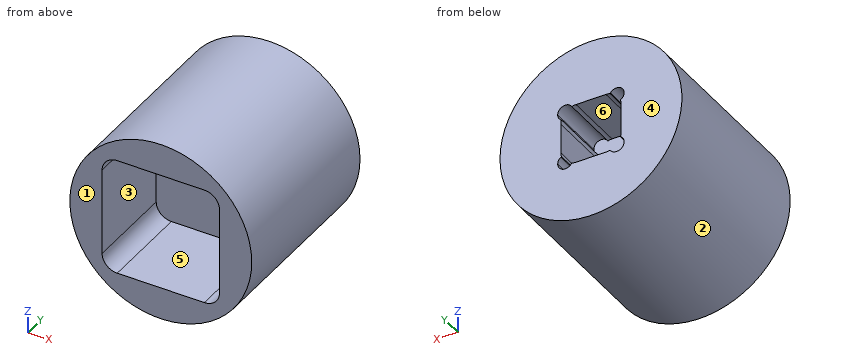
```python
from build123d import *

# Parameters (mm, degrees)
SKETCH1_R           = 19.05
BOSS_EXTRUDE1_DEPTH = 19.05
SKETCH2_W           = 12.6111
SKETCH2_H           = 12.6111
CUT_EXTRUDE1_DEPTH  = 12.7
CUT_EXTRUDE2_DEPTH  = 19.05
FILLET1_R           = 3.175
CUT_EXTRUDE3_DEPTH  = 12.7


with BuildPart() as part:
    # Sketch1 → Boss-Extrude1 (new body, symmetric)
    with BuildSketch(Plane(origin=(0, 0, 0), x_dir=(1, 0, 0), z_dir=(0, 1, 0))):
        Circle(SKETCH1_R)
    extrude(amount=BOSS_EXTRUDE1_DEPTH, both=True)

    # Sketch2 → Cut-Extrude1 (cut)
    with BuildSketch(Plane(origin=(0, 19.05, 0), x_dir=(1, 0, 0), z_dir=(0, 1, 0))):
        Rectangle(SKETCH2_W, SKETCH2_H)
    extrude(amount=-CUT_EXTRUDE1_DEPTH, mode=Mode.SUBTRACT)

    # Sketch3 → Cut-Extrude2 (cut)
    with BuildSketch(Plane.XZ.offset(19.05)):
        with BuildLine():
            Line((9.12495, 12.29995), (-9.12495, 12.29995))
            ThreePointArc((-9.12495, 12.29995), (-11.37001403, 11.37001403), (-12.29995, 9.12495))
            Line((-12.29995, 9.12495), (-12.29995, -9.12495))
            ThreePointArc((-12.29995, -9.12495), (-11.37001403, -11.37001403), (-9.12495, -12.29995))
            Line((-9.12495, -12.29995), (9.12495, -12.29995))
            ThreePointArc((9.12495, -12.29995), (11.37001403, -11.37001403), (12.29995, -9.12495))
            Line((12.29995, -9.12495), (12.29995, 9.12495))
            ThreePointArc((12.29995, 9.12495), (11.37001403, 11.37001403), (9.12495, 12.29995))
        make_face()
    extrude(amount=-CUT_EXTRUDE2_DEPTH, mode=Mode.SUBTRACT)

    # Fillet1
    fillet1_edges = [part.edges().sort_by_distance(p)[0] for p in [
        (-6.30555, 12.7, 6.30555),
        (-6.30555, 12.7, -6.30555),
        (6.30555, 12.7, -6.30555),
        (6.30555, 12.7, 6.30555),
    ]]
    fillet(fillet1_edges, radius=FILLET1_R)

    # Sketch4 → Cut-Extrude3 (cut)
    with BuildSketch(Plane(origin=(0, 19.05, 0), x_dir=(1, 0, 0), z_dir=(0, 1, 0))):
        with BuildLine():
            ThreePointArc((4.008094076, 6.181867977), (4.253082015, 4.253082015), (6.181867977, 4.008094076))
            ThreePointArc((6.181867977, 4.008094076), (5.37561403, 5.37561403), (4.008094076, 6.181867977))
        make_face()
        with BuildLine():
            ThreePointArc((6.181867977, 4.008094076), (6.244651028, 4.047106994), (6.30555, 4.089000125))
            Line((6.30555, 4.089000125), (6.30555, 6.30555))
            Line((6.30555, 6.30555), (4.089000125, 6.30555))
            ThreePointArc((4.089000125, 6.30555), (4.047106994, 6.244651028), (4.008094076, 6.181867977))
            ThreePointArc((4.008094076, 6.181867977), (5.37561403, 5.37561403), (6.181867977, 4.008094076))
        make_face()
        with BuildLine():
            Line((6.30555, 6.30555), (6.30555, 4.089000125))
            ThreePointArc((6.30555, 4.089000125), (6.789196289, 4.653158877), (6.96311403, 5.37561403))
            ThreePointArc((6.96311403, 5.37561403), (5.864314693, 6.886020569), (4.089000125, 6.30555))
            Line((4.089000125, 6.30555), (6.30555, 6.30555))
        make_face()
        with BuildLine():
            ThreePointArc((-4.008094076, 6.181867977), (-5.37561403, 5.37561403), (-6.181867977, 4.008094076))
            ThreePointArc((-6.181867977, 4.008094076), (-4.588140821, 3.997193849), (-3.78811403, 5.37561403))
            ThreePointArc((-3.78811403, 5.37561403), (-3.844096127, 5.793476641), (-4.008094076, 6.181867977))
        make_face()
        with BuildLine():
            Line((-6.30555, 6.30555), (-6.30555, 4.089000125))
            ThreePointArc((-6.30555, 4.089000125), (-6.244651028, 4.047106994), (-6.181867977, 4.008094076))
            ThreePointArc((-6.181867977, 4.008094076), (-5.37561403, 5.37561403), (-4.008094076, 6.181867977))
            ThreePointArc((-4.008094076, 6.181867977), (-4.047106994, 6.244651028), (-4.089000125, 6.30555))
            Line((-4.089000125, 6.30555), (-6.30555, 6.30555))
        make_face()
        with BuildLine():
            ThreePointArc((-4.089000125, 6.30555), (-6.498146045, 6.498146045), (-6.30555, 4.089000125))
            Line((-6.30555, 4.089000125), (-6.30555, 6.30555))
            Line((-6.30555, 6.30555), (-4.089000125, 6.30555))
        make_face()
        with BuildLine():
            ThreePointArc((-6.30555, -4.089000125), (-6.498146045, -6.498146045), (-4.089000125, -6.30555))
            Line((-4.089000125, -6.30555), (-6.30555, -6.30555))
            Line((-6.30555, -6.30555), (-6.30555, -4.089000125))
        make_face()
        with BuildLine():
            Line((-6.30555, -6.30555), (-4.089000125, -6.30555))
            ThreePointArc((-4.089000125, -6.30555), (-4.047106994, -6.244651028), (-4.008094076, -6.181867977))
            ThreePointArc((-4.008094076, -6.181867977), (-5.37561403, -5.37561403), (-6.181867977, -4.008094076))
            ThreePointArc((-6.181867977, -4.008094076), (-6.244651028, -4.047106994), (-6.30555, -4.089000125))
            Line((-6.30555, -4.089000125), (-6.30555, -6.30555))
        make_face()
        with BuildLine():
            ThreePointArc((-6.181867977, -4.008094076), (-5.37561403, -5.37561403), (-4.008094076, -6.181867977))
            ThreePointArc((-4.008094076, -6.181867977), (-3.844096127, -5.793476641), (-3.78811403, -5.37561403))
            ThreePointArc((-3.78811403, -5.37561403), (-4.588140821, -3.997193849), (-6.181867977, -4.008094076))
        make_face()
        with BuildLine():
            ThreePointArc((6.181867977, -4.008094076), (4.253082015, -4.253082015), (4.008094076, -6.181867977))
            ThreePointArc((4.008094076, -6.181867977), (5.37561403, -5.37561403), (6.181867977, -4.008094076))
        make_face()
        with BuildLine():
            ThreePointArc((4.008094076, -6.181867977), (4.047106994, -6.244651028), (4.089000125, -6.30555))
            Line((4.089000125, -6.30555), (6.30555, -6.30555))
            Line((6.30555, -6.30555), (6.30555, -4.089000125))
            ThreePointArc((6.30555, -4.089000125), (6.244651028, -4.047106994), (6.181867977, -4.008094076))
            ThreePointArc((6.181867977, -4.008094076), (5.37561403, -5.37561403), (4.008094076, -6.181867977))
        make_face()
        with BuildLine():
            Line((6.30555, -6.30555), (4.089000125, -6.30555))
            ThreePointArc((4.089000125, -6.30555), (5.864314693, -6.886020569), (6.96311403, -5.37561403))
            ThreePointArc((6.96311403, -5.37561403), (6.789196289, -4.653158877), (6.30555, -4.089000125))
            Line((6.30555, -4.089000125), (6.30555, -6.30555))
        make_face()
    extrude(amount=-CUT_EXTRUDE3_DEPTH, mode=Mode.SUBTRACT)


solid = part.part
```
Here's how the part is built. I have some questions about the finished solid (model axes, mm). Face numbers are marked on the shaded views. A direction names the side the tool comes from. Coordinates: 2 decimals unless noted, no trailing zeros. Order: outer loops, then holes, each group sorted by start corner. A loop starts at its lowest first (then second) coordinate and runs counter-clockwise, first axis right, second up. Notation, with made-up numbers: M 14,-35 L 21,-35 A19 ccw 21,-7 Z; hole C -27.75,17 d7. An arc over 180 degrees is marked long. Answer as a JSON object with one key per item and string values. Group by question number.
(1) Suppose I cut it at A-A, the plane y = -4. Please give me the cut outline in (x, z) (3 decimals).
(2) Suppose I cut it at C-C, the plane z = 0. Please give me the cut outline in (x, y).
(3) Which directions (+Z, -Z, +X, -X, +Y, -Y) give clear straight access to the entire face, cutting with the end or side of a thin tool? Please do the marked faces 4, 5 and 6.
(4) For pin 1 (1.9 mm diameter, centred on x = -5.38, z = -5.38, fed in from +Y); pin 2 (7 mm diameter, centred on x = -1, y = 12.5, fed in from -Z); pin 3 (5.5 mm diameter, centred on x = -2, y = -14, fed in from +Z), each with a flat end and sliding along its axis, tell me the tip position at first contact or that it passes through.
(5) I need wall thicknesses on probe 1 along Z at (x, y) = (2.5, 17); probe 2 along Z at (x, y) = (3.5, -13.5); probe 3 along Y at (x, z) = (-1, 8). Which ranges of each line are inside material? Lowest first, please.
(6) Suppose I cut it at B-B, the plane x = 0. Please give me the cut outline in (y, z), then the cut area to 3 significant figures.
(7) If we mould it in two halves opening along X, with no side actions, what happens to the marked faces 1, 2 and 3? For each: released by +X, released by -X, zero draft, split by the parting line, or undercut.
Values found:
{
 "1": {"outline": "C 0,0 d38.1; hole M -12.3,-9.125 A3.175 ccw -9.125,-12.3 L 9.125,-12.3 A3.175 ccw 12.3,-9.125 L 12.3,9.125 A3.175 ccw 9.125,12.3 L -9.125,12.3 A3.175 ccw -12.3,9.125 Z"},
 "2": {"outline": "M -19.05,-19.05 L -12.3,-19.05 L -12.3,0 L 12.3,0 L 12.3,-19.05 L 19.05,-19.05 L 19.05,19.05 L 6.31,19.05 L 6.31,6.35 L -6.31,6.35 L -6.31,19.05 L -19.05,19.05 Z"},
 "3": {"face 4": "+Z, -Z, +X, -X, +Y", "face 5": "-Y", "face 6": "+Y"},
 "4": {"pin 1": "stops at y = 6.35", "pin 2": "stops at z = -19.05", "pin 3": "stops at z = 19.05"},
 "5": {"probe 1": "z = -18.89 to -6.31, 6.31 to 18.89", "probe 2": "z = -18.73 to -12.3, 12.3 to 18.73", "probe 3": "y = 0 to 19.05"},
 "6": {"outline": "M -19.05,-19.05 L 19.05,-19.05 L 19.05,-6.31 L 6.35,-6.31 L 6.35,6.31 L 19.05,6.31 L 19.05,19.05 L -19.05,19.05 L -19.05,12.3 L 0,12.3 L 0,-12.3 L -19.05,-12.3 Z", "area": "823 mm^2"},
 "7": {"face 1": "zero draft", "face 2": "split by the parting line", "face 3": "undercut"}
}
